Design review of the part built by this model. Coordinates are the model's own, in mm. Face numbers are marked on the shaded views. Coordinates: 2 decimals unless noted, no trailing zeros. Write each loop counter-clockwise with the first axis right and the second up, starting at its lowest first coordinate (ties: lowest second). Pieces come first, ordered by that corner, then holes. Notation, with made-up numbers: (-35.75, 14.25) - (-21.75, 14.25) arc R25 ccw to (-21.75, 38.25) - close; hole circle Ø10 at (73.25, -0.5). An arc over 180 degrees is marked (long way). Answer as a JSON object with one key per item and string values.
```python
from build123d import *

# Parameters (mm, degrees)
SKETCH2_W           = 124
SKETCH2_H           = 62
SKETCH2_R           = 1.55
SKETCH2_W_2         = 26.6
SKETCH2_H_2         = 14.6
SKETCH2_R_2         = 8.3
SKETCH2_R_3         = 8.2
BOSS_EXTRUDE1_DEPTH = 4
CHAMFER1_SIZE       = 1.5
CHAMFER2_SIZE       = 1
SKETCH2_3_R         = 0.8
BOSS_EXTRUDE2_DEPTH = 3.5
FILLET1_R           = 0.8
CUT_EXTRUDE1_START  = 3
SKETCH2_4_W         = 28
SKETCH2_4_H         = 28.35
SKETCH2_4_R         = 0.8
SKETCH2_4_W_2       = 26.6
SKETCH2_4_H_2       = 14.6
CUT_EXTRUDE1_DEPTH  = 3
CHAMFER3_SIZE       = 1


with BuildPart() as part:
    # Sketch2 → Boss-Extrude1 (new body)
    with BuildSketch(Plane(origin=(0, 0, 0), x_dir=(1, 0, 0), z_dir=(0, 1, 0))):
        with Locations((62, 31)):
            Rectangle(SKETCH2_W, SKETCH2_H)
        with Locations(Location((4.5, 4.5, 0), (0, 0, 270))):
            Circle(SKETCH2_R, mode=Mode.SUBTRACT)
        with Locations(Location((119.5, 4.5, 0), (0, 0, 270))):
            Circle(SKETCH2_R, mode=Mode.SUBTRACT)
        with Locations(Location((4.5, 57.5, 0), (0, 0, 270))):
            Circle(SKETCH2_R, mode=Mode.SUBTRACT)
        with Locations(Location((119.5, 57.5, 0), (0, 0, 270))):
            Circle(SKETCH2_R, mode=Mode.SUBTRACT)
        with Locations((28.239743387, 41.89740921)):
            Rectangle(SKETCH2_W_2, SKETCH2_H_2, mode=Mode.SUBTRACT)
        with Locations(Location((102.593331931, 31, 0), (0, 0, 270))):
            Circle(SKETCH2_R_2, mode=Mode.SUBTRACT)
        with Locations(Location((75.171087178, 14.839562505, 0), (0, 0, 270))):
            Circle(SKETCH2_R_3, mode=Mode.SUBTRACT)
        with BuildLine():
            ThreePointArc((66.375, 36.123659504), (56.075, 40.119282109), (66.375, 44.114904714))
            Line((66.375, 44.114904714), (66.375, 36.123659504))
        make_face(mode=Mode.SUBTRACT)
        with Locations(Location((48.846547615, 14.839562505, 0), (0, 0, 270))):
            Circle(SKETCH2_R_3, mode=Mode.SUBTRACT)
        with Locations(Location((23.171087178, 14.839562505, 0), (0, 0, 270))):
            Circle(SKETCH2_R_3, mode=Mode.SUBTRACT)
    extrude(amount=BOSS_EXTRUDE1_DEPTH)

    # Chamfer1
    chamfer1_edges = [part.edges().sort_by_distance(p)[0] for p in [
        (62, 4, 0),
        (124, 4, -31),
        (62, 4, -62),
        (0, 4, -31),
    ]]
    chamfer(chamfer1_edges, length=CHAMFER1_SIZE)

    # Chamfer2
    chamfer2_edges = [part.edges().sort_by_distance(p)[0] for p in [
        (119.5, 0, -59.05),
        (4.5, 4, -6.05),
        (119.5, 4, -59.05),
        (119.5, 4, -6.05),
        (4.5, 4, -59.05),
    ]]
    chamfer(chamfer2_edges, length=CHAMFER2_SIZE)

    # Sketch2<3> → Boss-Extrude2 (add)
    with BuildSketch(Plane(origin=(0, 0, 0), x_dir=(1, 0, 0), z_dir=(0, 1, 0))):
        with Locations(Location((16.679743387, 28.409287577, 0), (0, 0, 270))):
            Circle(SKETCH2_3_R)
        with Locations(Location((16.679743387, 51.709287577, 0), (0, 0, 270))):
            Circle(SKETCH2_3_R)
        with Locations(Location((39.799743387, 28.409287577, 0), (0, 0, 270))):
            Circle(SKETCH2_3_R)
        with Locations(Location((39.799743387, 51.709287577, 0), (0, 0, 270))):
            Circle(SKETCH2_3_R)
    extrude(amount=-BOSS_EXTRUDE2_DEPTH)

    # Fillet1
    fillet1_edges = [part.edges().sort_by_distance(p)[0] for p in [
        (39.799743387, -3.5, -29.209287577),
        (39.799743387, -3.5, -52.509287577),
        (16.679743387, -3.5, -29.209287577),
        (16.679743387, -3.5, -52.509287577),
    ]]
    fillet(fillet1_edges, radius=FILLET1_R)

    # Sketch2<4> → Cut-Extrude1 (cut)
    with BuildSketch(Plane(origin=(0, 0, 0), x_dir=(1, 0, 0), z_dir=(0, 1, 0)).offset(CUT_EXTRUDE1_START)):
        with Locations((28.239743387, 39.62240921)):
            Rectangle(SKETCH2_4_W, SKETCH2_4_H)
        with Locations(Location((16.679743387, 51.709287577, 0), (0, 0, 270))):
            Circle(SKETCH2_4_R, mode=Mode.SUBTRACT)
        with Locations(Location((16.679743387, 28.409287577, 0), (0, 0, 270))):
            Circle(SKETCH2_4_R, mode=Mode.SUBTRACT)
        with Locations(Location((39.799743387, 28.409287577, 0), (0, 0, 270))):
            Circle(SKETCH2_4_R, mode=Mode.SUBTRACT)
        with Locations(Location((39.799743387, 51.709287577, 0), (0, 0, 270))):
            Circle(SKETCH2_4_R, mode=Mode.SUBTRACT)
        with Locations((28.239743387, 41.89740921)):
            Rectangle(SKETCH2_4_W_2, SKETCH2_4_H_2, mode=Mode.SUBTRACT)
    extrude(amount=-CUT_EXTRUDE1_DEPTH, mode=Mode.SUBTRACT)

    # Chamfer3
    chamfer3_edges = [part.edges().sort_by_distance(p)[0] for p in [
        (28.239743387, 4, -34.59740921),
        (41.539743387, 4, -41.89740921),
        (14.939743387, 4, -41.89740921),
        (28.239743387, 4, -49.19740921),
    ]]
    chamfer(chamfer3_edges, length=CHAMFER3_SIZE - 0.0001)  # a hair under: the kernel refuses the full size


solid = part.part
```
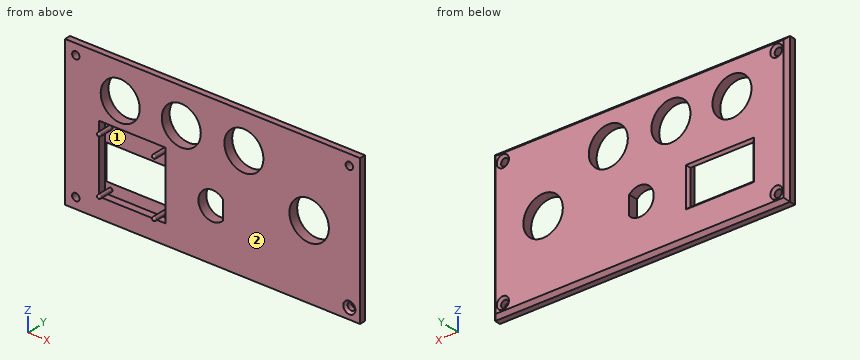
(1) For pin 1 (13 mm diameter, centred on x = 23.17, z = -14.84, fed in from -Y); pin 2 (1 mm diameter, centred on x = 84.5, z = -11.5, fed in from -Y); pin 3 (14 mm diameter, centred on x = 32.5, z = -40.5, fed in from -Y), all flat-tipped, find the tip position at first contact; note any pin that passes through.
Solved:
{"pin 1": "passes through", "pin 2": "stops at y = 0", "pin 3": "stops at y = 3"}
(2) The part is to be moulded in two halves that separate along Z. For the marked faces 1 and 2, say which applies: pulls with the +Z half, pulls with the -Z half, needs draft (parallel to the pull), parting line crosses it, or undercut.
Solved:
{"face 1": "undercut", "face 2": "needs draft"}
(3) Take a section at C-C, the plane z = -4.5. Write out the cut boundary in (x, y).
Solved:
{"outline": "(0, 0) - (2.95, 0) - (2.95, 3) - (1.95, 4) - (1.5, 4) - (0, 2.5) - close; (6.05, 0) - (117.95, 0) - (117.95, 3) - (116.95, 4) - (7.05, 4) - (6.05, 3) - close; (121.05, 0) - (124, 0) - (124, 2.5) - (122.5, 4) - (122.05, 4) - (121.05, 3) - close"}
(4) Take a section at B-B, the plane x = 4.5. Write out the cut boundary in (y, z).
Solved:
{"outline": "(0, -62) - (2.5, -62) - (4, -60.5) - (4, -60.05) - (3, -59.05) - (0, -59.05) - close; (0, -55.95) - (3, -55.95) - (4, -54.95) - (4, -7.05) - (3, -6.05) - (0, -6.05) - close; (0, -2.95) - (3, -2.95) - (4, -1.95) - (4, -1.5) - (2.5, 0) - (0, 0) - close"}
(5) To check wall thickness, follow line 1 (X direction, y = 2.2, z = -31); line 2 (X direction, y = 1.35, z = -57.5); line 3 (X direction, y = 1, z = -49.5). State the ranges of each line that lie inside material, in increasing order. Write a range as from..to.
Solved:
{"line 1": "x = 0..14.24, 42.24..94.29, 110.89..124", "line 2": "x = 0..2.95, 6.05..117.95, 121.05..124", "line 3": "x = 0..14.24, 42.24..124"}
(6) Take a section at A-A, the plane z = -31. Write out the cut boundary in (x, y).
Solved:
{"outline": "(0, 0) - (14.24, 0) - (14.24, 3) - (42.24, 3) - (42.24, 0) - (94.29, 0) - (94.29, 4) - (1.5, 4) - (0, 2.5) - close; (110.89, 0) - (124, 0) - (124, 2.5) - (122.5, 4) - (110.89, 4) - close"}
